Part model, mm, in its own coordinate system. A direction names the side the tool comes from. Coordinates: 2 decimals unless noted, no trailing zeros.
from build123d import *

# Parameters (mm, degrees)
BOSS_EXTRUDE1_DEPTH      = 2
BOSS_EXTRUDE1_DEPTH_BACK = 2
SKETCH3_R                = 15
BOSS_EXTRUDE3_DEPTH      = 2
BOSS_EXTRUDE3_DEPTH_BACK = 2
SKETCH12_R               = 10
BOSS_EXTRUDE4_DEPTH      = 16
CUT_EXTRUDE1_DEPTH       = 57.031941152
CUT_EXTRUDE1_DEPTH_BACK  = 57.031941152
SKETCH7_R                = 4.1
SKETCH13_W               = 5.45
SKETCH13_H               = 2.3
CUT_EXTRUDE2_DEPTH       = 4
CUT_EXTRUDE3_DEPTH       = 6
CUT_EXTRUDE3_DEPTH_BACK  = 4
SKETCH14_R               = 1.5
CUT_EXTRUDE4_DEPTH       = 2.3


with BuildPart() as part:
    # Sketch2 → Revolve1 (revolve)
    with BuildSketch(Plane(origin=(0, 0, 0), x_dir=(0, 0, -1), z_dir=(1, 0, 0)), mode=Mode.PRIVATE) as revolve1_sk:
        Polygon((-9, 35.970899576), (9, 35.970899576), (9, 37.970899576), (11, 37.970899576), (11, 33.970899576), (-11, 33.970899576), (-11, 37.970899576), (-9, 37.970899576), align=None)
    revolve(revolve1_sk.sketch.rotate(Axis((0, 0, 10), (0, 0, -1)), 90), axis=Axis((0, 0, 10), (0, 0, -1)))



with BuildPart() as body_2:
    # Sketch3 → Boss-Extrude1 (new, two sides: drawn at the far end of the back side and taken through both)
    with BuildSketch(Plane.XY.offset(-BOSS_EXTRUDE1_DEPTH_BACK)):
        Circle(SKETCH3_R)
    extrude(amount=BOSS_EXTRUDE1_DEPTH + BOSS_EXTRUDE1_DEPTH_BACK)


with BuildPart() as part_1:
    add(part.part)

    add(body_2.part)  # Boss-Extrude3 merges body 2
    # Sketch11 → Boss-Extrude3 (add, two sides: drawn at the far end of the back side and taken through both)
    with BuildSketch(Plane.XY.offset(-BOSS_EXTRUDE3_DEPTH_BACK)):
        with BuildLine():
            Line((5, 33.970899576), (-5, 33.970899576))
            add(Edge.make_bspline(
                [(-5, 33.970899576), (-3.602966052, 22.002598894), (-5.219370498, 14.062651656)],
                knots=[0, 0, 0, 0.277878322, 0.277878322, 0.277878322], degree=2))
            add(Edge.make_bspline(
                [(-5.219370498, 14.062651656), (-3.623415853, 14.571458155), (-2.092021841, 14.791258924)],
                knots=[0, 0, 0, 0.220994238, 0.220994238, 0.220994238], degree=2))
            add(Edge.make_bspline(
                [(-2.092021841, 14.791258924), (0.275566205, 15.158843416), (2.712697031, 14.915974307), (5.219370636, 14.062651605)],
                knots=[0.31222072, 0.31222072, 0.31222072, 0.31222072, 0.753229942, 0.753229942, 0.753229942, 0.753229942], degree=3))
            add(Edge.make_bspline(
                [(5, 33.970899576), (3.602966194, 22.002598839), (5.219370636, 14.062651605)],
                knots=[0, 0, 0, 0.277878321, 0.277878321, 0.277878321], degree=2))
        make_face()
        with BuildLine():
            Line((33.853330378, 5.742302702), (30.763160434, 15.252867865))
            add(Edge.make_bspline(
                [(30.763160434, 15.252867865), (19.812337313, 10.225801321), (11.76150231, 9.309514671)],
                knots=[0, 0, 0, 0.277878322, 0.277878322, 0.277878322], degree=2))
            add(Edge.make_bspline(
                [(11.76150231, 9.309514671), (12.738583154, 7.948901461), (13.420852883, 6.56038138)],
                knots=[0, 0, 0, 0.220994238, 0.220994238, 0.220994238], degree=2))
            add(Edge.make_bspline(
                [(13.420852883, 6.56038138), (14.50207145, 4.422261196), (15.024204045, 2.029361361), (14.987250672, -0.618318123)],
                knots=[0.31222072, 0.31222072, 0.31222072, 0.31222072, 0.753229942, 0.753229942, 0.753229942, 0.753229942], degree=3))
            add(Edge.make_bspline(
                [(33.853330378, 5.742302702), (22.039092786, 3.372552484), (14.987250672, -0.618318123)],
                knots=[0, 0, 0, 0.277878321, 0.277878321, 0.277878321], degree=2))
        make_face()
        with BuildLine():
            Line((15.922508806, -30.421961333), (24.01267875, -24.54410881))
            add(Edge.make_bspline(
                [(24.01267875, -24.54410881), (15.847663908, -15.682706115), (12.488378684, -8.309055171)],
                knots=[0, 0, 0, 0.277878322, 0.277878322, 0.277878322], degree=2))
            add(Edge.make_bspline(
                [(12.488378684, -8.309055171), (11.496293211, -9.658766879), (10.386565081, -10.736720252)],
                knots=[0, 0, 0, 0.220994238, 0.220994238, 0.220994238], degree=2))
            add(Edge.make_bspline(
                [(10.386565081, -10.736720252), (8.687206859, -12.42573569), (6.572771723, -13.661760011), (4.043259677, -14.444793221)],
                knots=[0.31222072, 0.31222072, 0.31222072, 0.31222072, 0.753229942, 0.753229942, 0.753229942, 0.753229942], degree=3))
            add(Edge.make_bspline(
                [(15.922508806, -30.421961333), (10.017942228, -19.918246775), (4.043259677, -14.444793221)],
                knots=[0, 0, 0, 0.277878321, 0.277878321, 0.277878321], degree=2))
        make_face()
        with BuildLine():
            Line((-24.01267875, -24.54410881), (-15.922508806, -30.421961333))
            add(Edge.make_bspline(
                [(-15.922508806, -30.421961333), (-10.017942375, -19.918246736), (-4.043259819, -14.444793181)],
                knots=[0, 0, 0, 0.277878322, 0.277878322, 0.277878322], degree=2))
            add(Edge.make_bspline(
                [(-4.043259819, -14.444793181), (-5.633483205, -13.918347682), (-7.001602636, -13.196039424)],
                knots=[0, 0, 0, 0.220994238, 0.220994238, 0.220994238], degree=2))
            add(Edge.make_bspline(
                [(-7.001602636, -13.196039424), (-9.133082344, -12.101788187), (-10.96200772, -10.472793393), (-12.488378766, -8.309055048)],
                knots=[0.31222072, 0.31222072, 0.31222072, 0.31222072, 0.753229942, 0.753229942, 0.753229942, 0.753229942], degree=3))
            add(Edge.make_bspline(
                [(-24.01267875, -24.54410881), (-15.847663991, -15.682705988), (-12.488378766, -8.309055048)],
                knots=[0, 0, 0, 0.277878321, 0.277878321, 0.277878321], degree=2))
        make_face()
        with BuildLine():
            Line((-30.763160434, 15.252867865), (-33.853330378, 5.742302702))
            add(Edge.make_bspline(
                [(-33.853330378, 5.742302702), (-22.039092794, 3.372552636), (-14.987250678, -0.618317975)],
                knots=[0, 0, 0, 0.277878322, 0.277878322, 0.277878322], degree=2))
            add(Edge.make_bspline(
                [(-14.987250678, -0.618317975), (-14.977977306, 1.056754944), (-14.713793486, 2.581119372)],
                knots=[0, 0, 0, 0.220994238, 0.220994238, 0.220994238], degree=2))
            add(Edge.make_bspline(
                [(-14.713793486, 2.581119372), (-14.33176217, 4.946419265), (-13.347665078, 7.189217736), (-11.761502219, 9.309514786)],
                knots=[0.31222072, 0.31222072, 0.31222072, 0.31222072, 0.753229942, 0.753229942, 0.753229942, 0.753229942], degree=3))
            add(Edge.make_bspline(
                [(-30.763160434, 15.252867865), (-19.812337217, 10.225801439), (-11.761502219, 9.309514786)],
                knots=[0, 0, 0, 0.277878321, 0.277878321, 0.277878321], degree=2))
        make_face()
    extrude(amount=BOSS_EXTRUDE3_DEPTH + BOSS_EXTRUDE3_DEPTH_BACK)

    # Sketch12 → Boss-Extrude4 (add)
    with BuildSketch(Plane.XY):
        Circle(SKETCH12_R)
    extrude(amount=BOSS_EXTRUDE4_DEPTH)

    # Sketch7 → Cut-Extrude1 (cut, two sides: drawn at the far end of the back side and taken through both)
    with BuildSketch(Plane.XY.offset(-CUT_EXTRUDE1_DEPTH_BACK)):
        Circle(SKETCH7_R)
    extrude(amount=CUT_EXTRUDE1_DEPTH + CUT_EXTRUDE1_DEPTH_BACK, mode=Mode.SUBTRACT)

    # Sketch13 → Cut-Extrude2 (cut)
    with BuildSketch(Plane.XY.offset(16)):
        with Locations((0, 6.614053633)):
            Rectangle(SKETCH13_W, SKETCH13_H)
    extrude(amount=-CUT_EXTRUDE2_DEPTH, mode=Mode.SUBTRACT)

    # Sketch14 → Cut-Extrude3 (cut, two sides: drawn at the far end of the back side and taken through both)
    with BuildSketch(Plane(origin=(0, 5.464053633, 0), x_dir=(1, 0, 0), z_dir=(0, 1, 0)).offset(-CUT_EXTRUDE3_DEPTH_BACK)):
        with Locations((0, -12)):
            Circle(SKETCH14_R)
    extrude(amount=CUT_EXTRUDE3_DEPTH + CUT_EXTRUDE3_DEPTH_BACK, mode=Mode.SUBTRACT)

    # Sketch16 → Cut-Extrude4 (cut)
    with BuildSketch(Plane(origin=(0, 5.464053633, 0), x_dir=(1, 0, 0), z_dir=(0, 1, 0))):
        Polygon((0, -15.124596023), (2.705979533, -13.562298012), (2.705979533, -10.437701988), (0, -8.875403977), (-2.705979533, -10.437701988), (-2.705979533, -13.562298012), align=None)
    extrude(amount=CUT_EXTRUDE4_DEPTH, mode=Mode.SUBTRACT)


solid = part_1.part
Q1. Mould opens along Y. For faces 1 (the face through (-28, 20, -11)), 2 (the face through (-0.325, 8.868, 13.464)), 3 (the face through (-9, 12, 0)), 4 (the face through (-28.545, 21.888, -0.126)) say: pulls with the +Y half, pulls with the -Y half, needs draft (parallel to the pull), parting line crosses it, or undercut.
Results list:
face 1: needs draft
face 2: undercut
face 3: undercut
face 4: parting line crosses it
Q2. Which spindle directions (+Z, -Z, +X, -X, +Y, -Y) get a long thin tool onto all of the face, cutting with end or side? Do faces 5 (the face through (2, -5, -2)), 6 (the face through (14.25, -4.69, -0.03)), 7 (the face through (-23, 28, 9)), 8 (the face through (0, 5.464, 14)). Say none if no direction does.
Results list:
face 5: -Z
face 6: +Z, -Z
face 7: none
face 8: +Z
Q3. Pin check, flat tips, straight feed: pin 1 Ø5 at (y, z) = (12.5, 7) entering from +X; pin 2 Ø10 at (y, z) = (7.5, -3.5) entering from +X; pin 3 Ø5 at (x, y) = (-20, 22) entering from -Z; pin 4 Ø1.7 at (y, z) = (7, 11.5) entering from -X. Stop position of each tip, or through.
Results list:
pin 1: stops at x = 36.34
pin 2: stops at x = 35.88
pin 3: passes through
pin 4: stops at x = -37.44
Q4. Wall check: line 1 along Y through (x, z) = (0, -1.25); line 2 along Y through (x, z) = (0, 7.75); line 3 along Z through (x, y) = (0, 9). Give the ranges that are in metal, low to high.
Results list:
line 1: y = -35.97 to -33.97, -15 to -4.1, 4.1 to 35.97
line 2: y = -35.97 to -33.97, -10 to -4.1, 4.1 to 10, 33.97 to 35.97
line 3: z = -2 to 10.5, 13.5 to 16
Q5. Cut at A-A on x = 26. Count the separate pieces of the cut face and the enclosed holes in it, and give its area (3 significant figures).
Results list:
separate pieces: 3
enclosed holes: 0
area: 192 mm2
